Autodesk Inventor part; units mm, degrees
ref_plane "to_frame_XY" through (0, 0, 0) normal (0, 0, 1) x (1, 0, 0)
ref_plane "to_frame_YZ" through (0, 0, 0) normal (1, 0, 0) x (0, 1, 0)
ref_plane "to_frame_ZX" through (0, 0, 0) normal (0, 1, 0) x (0, 0, 1)
sketch "Sketch_5" plane through (0, 0, 0) normal (0, 0, 1) x (1, 0, 0)
  arc A0 (-10, 3.3) -> (-9.7, 3) centre (-9.7, 3.3) ccw
  line L0 (-9.7, 3) -> (-8, 3)
  line L1 (-8, 3) -> (-8, 6)
  line L2 (-8, 6) -> (-7.0607, 6)
  line L3 (-7.0607, 6) -> (-4, 2.9393)
  line L4 (-4, 2.9393) -> (-4, 0.3)
  line L5 (-4, 0.3) -> (-3.7, 0)
  line L6 (-3.7, 0) -> (-4, -0.3)
  line L7 (-4, -0.3) -> (-4, -2.9393)
  line L8 (-4, -2.9393) -> (-7.0607, -6)
  line L9 (-7.0607, -6) -> (-8, -6)
  line L10 (-8, -6) -> (-8, -3)
  line L11 (-8, -3) -> (-9.7, -3)
  arc A1 (-9.7, -3) -> (-10, -3.3) centre (-9.7, -3.3) ccw
  line L12 (-10, -3.3) -> (-10, -9)
  arc A2 (-10, -9) -> (-9, -10) centre (-9, -9) ccw
  line L13 (-9, -10) -> (-3.3, -10)
  arc A3 (-3.3, -10) -> (-3, -9.7) centre (-3.3, -9.7) ccw
  line L14 (-3, -9.7) -> (-3, -8)
  line L15 (-3, -8) -> (-6, -8)
  line L16 (-6, -8) -> (-6, -7.0607)
  line L17 (-6, -7.0607) -> (-2.9393, -4)
  line L18 (-2.9393, -4) -> (-0.3, -4)
  line L19 (-0.3, -4) -> (0, -3.7)
  line L20 (0, -3.7) -> (0.3, -4)
  line L21 (0.3, -4) -> (2.9393, -4)
  line L22 (2.9393, -4) -> (6, -7.0607)
  line L23 (6, -7.0607) -> (6, -8)
  line L24 (6, -8) -> (3, -8)
  line L25 (3, -8) -> (3, -9.7)
  arc A4 (3, -9.7) -> (3.3, -10) centre (3.3, -9.7) ccw
  line L26 (3.3, -10) -> (9, -10)
  arc A5 (9, -10) -> (10, -9) centre (9, -9) ccw
  line L27 (10, -9) -> (10, -3.3)
  arc A6 (10, -3.3) -> (9.7, -3) centre (9.7, -3.3) ccw
  line L28 (9.7, -3) -> (8, -3)
  line L29 (8, -3) -> (8, -6)
  line L30 (8, -6) -> (7.0607, -6)
  line L31 (7.0607, -6) -> (4, -2.9393)
  line L32 (4, -2.9393) -> (4, -0.3)
  line L33 (4, -0.3) -> (3.7, 0)
  line L34 (3.7, 0) -> (4, 0.3)
  line L35 (4, 0.3) -> (4, 2.9393)
  line L36 (4, 2.9393) -> (7.0607, 6)
  line L37 (7.0607, 6) -> (8, 6)
  line L38 (8, 6) -> (8, 3)
  line L39 (8, 3) -> (9.7, 3)
  arc A7 (9.7, 3) -> (10, 3.3) centre (9.7, 3.3) ccw
  line L40 (10, 3.3) -> (10, 9)
  arc A8 (10, 9) -> (9, 10) centre (9, 9) ccw
  line L41 (9, 10) -> (3.3, 10)
  arc A9 (3.3, 10) -> (3, 9.7) centre (3.3, 9.7) ccw
  line L42 (3, 9.7) -> (3, 8)
  line L43 (3, 8) -> (6, 8)
  line L44 (6, 8) -> (6, 7.0607)
  line L45 (6, 7.0607) -> (2.9393, 4)
  line L46 (2.9393, 4) -> (0.3, 4)
  line L47 (0.3, 4) -> (0, 3.7)
  line L48 (0, 3.7) -> (-0.3, 4)
  line L49 (-0.3, 4) -> (-2.9393, 4)
  line L50 (-2.9393, 4) -> (-6, 7.0607)
  line L51 (-6, 7.0607) -> (-6, 8)
  line L52 (-6, 8) -> (-3, 8)
  line L53 (-3, 8) -> (-3, 9.7)
  arc A10 (-3, 9.7) -> (-3.3, 10) centre (-3.3, 9.7) ccw
  line L54 (-3.3, 10) -> (-9, 10)
  arc A11 (-9, 10) -> (-10, 9) centre (-9, 9) ccw
  line L55 (-10, 9) -> (-10, 3.3)
  circle A12 centre (0, 0) radius 2.1
extrude "Extrusion1" add sketch "Sketch_5" against normal blind 30
ref_plane "to_frame_XY" through (0, 0, 0) normal (0, 0, 1) x (1, 0, 0)
ref_plane "to_frame_YZ" through (0, 0, 0) normal (1, 0, 0) x (0, 1, 0)
ref_plane "to_frame_ZX" through (0, 0, 0) normal (0, 1, 0) x (0, 0, 1)
properties part number "KHFS5-2020-1000"
Geometry check sheet. Reference: the model listing, model coordinates, mm. A direction names the side the tool comes from. Round coordinates to 2 decimals unless told otherwise and drop trailing zeros. Order: outer loops, then holes, each group sorted by start corner. A loop starts at its lowest first (then second) coordinate and runs counter-clockwise, first axis right, second up. Notation, with made-up numbers: (41.5, 24) - (88.5, 24) arc R21 ccw to (88.5, 46) - close; hole circle Ø3 at (-4.5, 13.5). An arc over 180 degrees is marked (long way). One line per question, with ' | ' between items. Start each with the question number.
(1) Sectioned sample at A-A on y = -5.5. Record the cut outline in (x, z), and give its area (3 significant figures).
(2) Sectioned sample at C-C on x = 5. Record the cut outline in (y, z), and give its area (3 significant figures).
(3) Depth check by flat-ended pin: pin 1 Ø1.3 at (x, z) = (1, -12.5) entering from +Y; pin 2 Ø1.3 at (y, z) = (1.5, -15) entering from -X; pin 3 Ø0.8 at (x, z) = (1.5, -21.5) entering from -Y. Enter the tip coordinate at first touch or a pass-through.
(4) Thickness scan on L1, parallel to Y at x = 8.5, z = -9.5; L2, parallel to X at y = -4.75, z = -25.75; L3, parallel to Y at x = 5, z = -3.25. Record the ranges inside material, lowest first. Write a range as [from, to].
(5) Sectioned sample at B-B on y = 0.75. Record the cut outline in (x, z), and give its area (3 significant figures).
(6) Access from +Z, -Z, +X, -X, +Y, -Y to the whole of each face (thin tool, end or side, straight path). Record for faces 4 (the flat face through (2, 4, -15)), 5 (the cylindrical face through (-9.699, 9.715, -14.79)), 6 (the flat face through (5.51, 4.45, -14.79)), 7 (the flat face through (-2, -4, -15)).
(7) Release check for a two-part mould opening along X. For faces 1 (the cylindrical face through (9.699, -9.715, -14.79)), 2 (the flat face through (9, 3, -15)), 3 (the flat face through (-8, 4, -15)) record: released by +X, released by -X, zero draft, split by the parting line, or undercut.
Conclusion:
1) outline: (-10, -30) - (-8, -30) - (-8, 0) - (-10, 0) - close; (-6.56, -30) - (-4.44, -30) - (-4.44, 0) - (-6.56, 0) - close; (4.44, -30) - (6.56, -30) - (6.56, 0) - (4.44, 0) - close; (8, -30) - (10, -30) - (10, 0) - (8, 0) - close | area: 247 mm2
2) outline: (-10, -30) - (-8, -30) - (-8, 0) - (-10, 0) - close; (-6.06, -30) - (-3.94, -30) - (-3.94, 0) - (-6.06, 0) - close; (3.94, -30) - (6.06, -30) - (6.06, 0) - (3.94, 0) - close; (8, -30) - (10, -30) - (10, 0) - (8, 0) - close | area: 247 mm2
3) pin 1: stops at y = 4 | pin 2: stops at x = -4 | pin 3: stops at y = -4
4) L1: y = [-10, -3], [3, 10] | L2: x = [-10, -8], [-5.81, -3.69], [3.69, 5.81], [8, 10] | L3: y = [-10, -8], [-6.06, -3.94], [3.94, 6.06], [8, 10]
5) outline: (-4, -30) - (-1.96, -30) - (-1.96, 0) - (-4, 0) - close; (1.96, -30) - (4, -30) - (4, 0) - (1.96, 0) - close | area: 122 mm2
6) face 4: +Z, -Z, +Y | face 5: +Z, -Z, -X, +Y | face 6: +Z, -Z | face 7: +Z, -Z, -Y
7) face 1: released by +X | face 2: zero draft | face 3: undercut
